Autodesk Inventor part; units mm, degrees
ref_plane "YZ Plane" through (0, 0, 0) normal (1, 0, 0) x (0, 1, 0)
ref_plane "XZ Plane" through (0, 0, 0) normal (0, 1, 0) x (-1, 0, 0)
ref_plane "XY Plane" through (0, 0, 0) normal (0, 0, 1) x (1, 0, 0)
sketch "Base" plane through (0, 0, 0) normal (0, 0, 1) x (1, 0, 0)
  line L0 (-15, -20) -> (15, -20)
  line L1 (15, -20) -> (15, 20)
  line L2 (15, 20) -> (-15, 20)
  line L3 (-15, 20) -> (-15, -20)
  line L4 (-15, -20) -> (15, 20) construction
  line L5 (15, -20) -> (-15, 20) construction
  circle A0 centre (0, 0) radius 11.125
  line L6 (-15, 20) -> (-11, 20)
  line L7 (-11, 20) -> (-11, 16)
  line L8 (-11, 16) -> (-15, 16)
  line L9 (-15, 16) -> (-15, 20)
  line L10 (-21, 0) -> (21, 0) construction
  line L11 (0, -28) -> (0, 28) construction
  line L12 (11, 20) -> (11, 16)
  line L13 (11, 16) -> (15, 16)
  line L14 (-11, -20) -> (-11, -16)
  line L15 (-11, -16) -> (-15, -16)
  line L16 (11, -16) -> (15, -16)
  line L17 (11, -20) -> (11, -16)
  dimension "d0" = 40
  dimension "d1" = 30
  dimension "d2" = 22.25
  dimension "d5" = 4
extrude "BaseFeature" add sketch "Base" along normal blind 10.6 contours L14 L15 L3 L8 L7 L2 L12 L13 L1 L16 L17 L0
fillet "BaseFilletsFeature" radius 1 11 edges at (-15, 16, 5.3) (-11, 20, 5.3) (11, 20, 5.3) (15, 16, 5.3) (-11, 16, 5.3) (-15, -16, 5.3) (-11, -16, 5.3) (-11, -20, 5.3) (11, -20, 5.3) (11, -16, 5.3) (15, -16, 5.3)
sketch "MountHoles" plane through (0, 0, 10.6) normal (0, 0, 1) x (1, 0, 0)
  line L0 (10, 20) -> (-10, 20)
  line L1 (-3, 20) -> (3, 20)
  line L2 (3, 20) -> (3, 19)
  line L3 (3, 19) -> (-3, 19)
  line L4 (-3, 19) -> (-3, 20)
  line L5 (-21, 0) -> (21, 0) construction
  line L6 (3, -20) -> (3, -19)
  line L7 (3, -19) -> (-3, -19)
  line L8 (-3, -19) -> (-3, -20)
  line L9 (-10, -20) -> (10, -20)
  circle A0 centre (0, 0) radius 11.125 construction
  circle A1 centre (0, 15) radius 2
  circle A2 centre (0, -15) radius 2
  line L10 (0, -28) -> (0, 28) construction
  point P0 (0, 20)
  dimension "d7" = 1
  dimension "d8" = 6
  dimension "d9" = 4
  dimension "d10" = 30
extrude "MountHolesFeature" cut sketch "MountHoles" against normal through all
sketch "Body" plane through (0, 0, 0) normal (0, 0, -1) x (-1, 0, 0)
  line L0 (15, 15) -> (0, 15)
  line L1 (0, 15) -> (0, -15)
  line L2 (0, -15) -> (15, -15)
  line L3 (15, -15) -> (15, 15)
  line L4 (15, 15) -> (15, -15)
  point P0 (0, 0)
  dimension "d13" = 15
extrude "BodyFeature" add sketch "Body" along normal blind 25
sketch "Chamfer" plane through (-15, -15, 10.6) normal (-1, 0, 0) x (0, 0, 1)
  line L0 (-10.6, 0) -> (-35.6, 0)
  line L1 (-10.6, 0) -> (-10.6, 2.3)
  line L2 (-10.6, 0) -> (-10.6, 30)
  line L3 (-10.6, 2.3) -> (-18.6, 0)
  line L4 (-42.72, 15) -> (7.12, 15) construction
  line L5 (-10.6, 30) -> (-10.6, 27.7)
  line L6 (-10.6, 27.7) -> (-18.6, 30)
  line L7 (-10.6, 30) -> (-35.6, 30)
  line L8 (-18.6, 30) -> (-18.6, 0) construction
  point P0 (-10.6, 15)
  dimension "d16" = 8
  dimension "d17" = 2.3
extrude "ChamferFeature" cut sketch "Chamfer" against normal through all
sketch "Terminals" plane through (0, 0, -25) normal (0, 0, -1) x (-1, 0, 0)
  line L0 (15, -15) -> (15, 15) construction
  line L1 (15, 15) -> (0, 15) construction
  line L2 (0, 15) -> (0, -15) construction
  line L3 (0, -15) -> (15, -15) construction
  line L4 (0, -15) -> (15, -15)
  line L5 (5.7, -15) -> (5.7, 15) construction
  line L6 (21, 0) -> (-21, 0) construction
  line L7 (5.7, -12.59) -> (8.87, -12.59)
  line L8 (8.87, -12.59) -> (8.87, -6.25) construction
  line L9 (8.87, -6.25) -> (5.7, -6.25)
  line L10 (5.7, -6.25) -> (5.7, -12.59)
  circle A0 centre (8.87, -9.42) radius 3.17
  line L11 (8.87, -9.42) -> (12.04, -9.42) construction
  line L12 (5.7, 12.59) -> (8.87, 12.59)
  line L13 (8.87, 6.25) -> (5.7, 6.25)
  line L14 (5.7, 6.25) -> (5.7, 12.59)
  circle A1 centre (8.87, 9.42) radius 3.17
  line L15 (5.7, -3.5) -> (9.4, -3.5)
  line L16 (9.4, -3.5) -> (9.4, 3.5)
  line L17 (9.4, 3.5) -> (5.7, 3.5)
  line L18 (5.7, 3.5) -> (5.7, -3.5)
  point P0 (0, 0)
  point P1 (5.7, 0)
  dimension "d20" = 6.34
  dimension "d21" = 5.7
  dimension "d22" = 12.5
  dimension "d23" = 3.7
  dimension "d24" = 7
extrude "TerminalsFeature" cut sketch "Terminals" against normal blind 10
sketch "Ring" plane through (0, 0, 10.6) normal (0, 0, 1) x (1, 0, 0)
  arc A0 (0, -11.125) -> (0, 11.125) centre (0, 0) ccw
  circle A1 centre (0, 0) radius 30
  circle A2 centre (0, 0) radius 11.25
  dimension "d27" = 60
  dimension "d28" = 22.5
extrude "RingFeature" add sketch "Ring" along normal blind 2.5
sketch "ButtonNeck" plane through (0, 0, 13.1) normal (0, 0, 1) x (1, 0, 0)
  arc A0 (0, -11.125) -> (0, 11.125) centre (0, 0) ccw
  circle A1 centre (0, 0) radius 13.5
  dimension "d31" = 27
extrude "ButtonNeckFeature" add sketch "ButtonNeck" along normal blind 11.5
sketch "ButtonBody" plane through (0, 0, 24.6) normal (0, 0, 1) x (1, 0, 0)
  circle A0 centre (0, 0) radius 11.25
  circle A1 centre (0, 0) radius 15
  dimension "d34" = 30
extrude "ButtonBodyFeature" add sketch "ButtonBody" along normal blind 13 contours A0 | A1
sketch "ButtonHead" plane through (0, 0, 0) normal (0, 1, 0) x (-1, 0, 0)
  line L0 (15, 37.6) -> (-15, 37.6)
  line L1 (-15, 37.6) -> (-19.5, 37.6)
  line L2 (-19.5, 37.6) -> (-19.5, 39.6)
  line L3 (-19.5, 39.6) -> (-20, 39.6)
  line L4 (-20, 39.6) -> (-20, 41.6)
  line L5 (-20, 41.6) -> (-19.5, 41.6)
  line L6 (-19.5, 41.6) -> (-19.5, 43.6)
  line L7 (-19.5, 43.6) -> (0, 43.6)
  line L8 (0, 43.6) -> (0, 37.6)
  line L9 (-20, 40.6) -> (0, 40.6) construction
  line L10 (0, -38.72) -> (0, 57.32)
  point P0 (0, 0)
  point P1 (-17.25, 37.6)
  dimension "d37" = 6
  dimension "d38" = 2
  dimension "d39" = 20
  dimension "d40" = 0.5
revolve "ButtonHeadFeature" add sketch "ButtonHead" angle 360 about axis through (0, 0, -10) along (0, 0, 1)
fillet "ButtonHeadFilletsFeature" radius 2 3 edges at (-15, 0, 37.6) (-19.5, 0, 37.6) (-19.5, 0, 43.6)
properties part number "E-Stop"
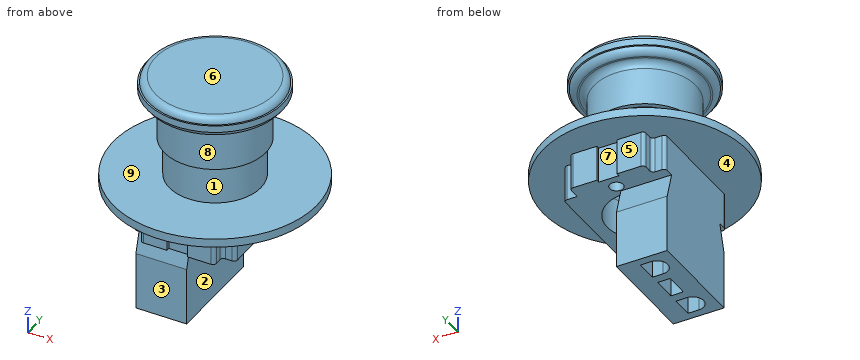
Model file for the job. Use its own axes, mm. Face numbers are marked on the shaded views. A direction names the side the tool comes from. Give positions to 0.01 mm unless a question says otherwise; leave off trailing zeros. Loops run counter-clockwise (first coordinate to the right, second up) from the corner with the lowest first, then second, coordinate; pieces in that order, holes last.
1) Pull direction Z, two halves, no side cores. Call the marked faces 6, 7, 8 and 9: +Z half, -Z half, draft (parallel to the pull), parting line (faces both ways), or undercut.
2) Tool access for the marked faces 1, 2, 3, 4 and 5: list every direction of +Z, -Z, +X, -X, +Y, -Y with a clear straight run to the whole face (end or side of a thin tool).
3) Saw through at D-D (x = 22). Write the cut outline in (y, z), plus the area to 3 significant figures.
4) Saw through at C-C (y = 23). Write the cut outline in (x, z).
5) Saw through at B-B (z = -20). Write the cut outline in (x, y).
6) Flat gauge pins, fed straight in: pin 1 Ø5.5 at (x, z) = (7.5, 7.5) entering from -Y; pin 2 Ø4 at (x, z) = (-19.5, 35.5) entering from -Y; pin 3 Ø1.5 at (x, z) = (3, 28) entering from -Y; pin 4 Ø6 at (x, y) = (-19.5, -10.5) entering from +Z. Where does each tip first touch, or does it go through?
7) Saw through at A-A (z = 3.5). Count the separate pieces of the cut face and the enclosed holes in it, plus the area to 3 significant figures.
8) Wall check: line 1 (Y direction, x = 0, z = 7) (3 decimals); line 2 (Z direction, x = -17.5, y = -1.5); line 3 (X direction, y = 0, z = 7.5) (3 decimals). Give the ranges that are in metal, low to high.
Answer block:
1. face 6: +Z half
1. face 7: draft
1. face 8: undercut
1. face 9: undercut
2. face 1: none
2. face 2: -Z, +X, +Y, -Y
2. face 3: -Z, +X, -X, -Y
2. face 4: -Z
2. face 5: -Z, +X, -X, +Y
3. outline: (-20.4, 10.6) - (20.4, 10.6) - (20.4, 13.1) - (-20.4, 13.1) - close
3. area: 102 mm2
4. outline: (-19.26, 10.6) - (19.26, 10.6) - (19.26, 13.1) - (-19.26, 13.1) - close
5. outline: (-15, -15) - (0, -15) - (0, 15) - (-15, 15) - close; hole (-9.4, -3.5) - (-5.7, -3.5) - (-5.7, 3.5) - (-9.4, 3.5) - close; hole (-8.87, -12.59) - (-5.7, -12.59) - (-5.7, -6.25) - (-8.87, -6.25) arc R3.17 ccw to start; hole (-8.87, 6.25) - (-5.7, 6.25) - (-5.7, 12.59) - (-8.87, 12.59) arc R3.17 ccw to start
6. pin 1: stops at y = -20
6. pin 2: passes through
6. pin 3: stops at y = -14.83
6. pin 4: stops at z = 42.73
7. separate pieces: 1
7. enclosed holes: 3
7. area: 709 mm2
8. line 1: y = -19 to -17, -13 to -11.125, 11.125 to 13, 17 to 19
8. line 2: z = 10.6 to 13.1, 37.6 to 43.6
8. line 3: x = -15 to -11.125, 11.125 to 15
